from build123d import *

# Parameters (mm, degrees)
EXTRUDE_1_DEPTH = 20
SKETCH_3_W      = 1.25
SKETCH_3_H      = 40.001


with BuildPart() as part:
    # 草图1 → 凸台-拉伸1 (new, symmetric)
    with BuildSketch(Plane(origin=(0, 0, 0), x_dir=(1, 0, 0), z_dir=(0, 1, 0))):
        Polygon((1.327905619, -2.3), (2.655811238, 0), (1.327905619, 2.3), (-1.327905619, 2.3), (-2.655811238, 0), (-1.327905619, -2.3), align=None)
    extrude(amount=EXTRUDE_1_DEPTH, both=True)

    # 草图3 → M3 螺纹孔1 (revolve, cut)
    with BuildSketch(Plane(origin=(0, 20, 0), x_dir=(0, 0, 1), z_dir=(1, 0, 0))):
        with Locations((0.625, 20.0005)):
            Rectangle(SKETCH_3_W, SKETCH_3_H)
    revolve(axis=Axis((0, 26.35, 0), (0, -1, 0)), mode=Mode.SUBTRACT)


solid = part.part
For this review, take the finished solid that the model builds, in its own axes (mm). Give positions to 0.01 mm unless a question says otherwise; leave off trailing zeros. Loops run counter-clockwise (first coordinate to the right, second up) from the corner with the lowest first, then second, coordinate; pieces in that order, holes last.
Item 1: Take a section at C-C, the plane z = 0.4. State the section outline as (x, y) points.
Item 2: Take a section at D-D, the plane x = 2.3. State the section outline as (y, z) points, and give its area (3 significant figures).
Item 3: Draft analysis for pull direction X (two halves, no side actions). For faces 1 (the flat face through (0, 0, 2.3)), 2 (the flat face through (-1.98, 0.28, -1.17)), 3 (the flat face through (1.98, 0.28, 1.17)), 4 (the cylindrical face through (1.22, -0.28, -0.27)), state which applies: +X half, -X half, draft (parallel to the pull), parting line (faces both ways), or undercut.
Item 4: Insertion check: pin 1 (1.5 mm diameter, centred on y = -3, z = 1, fed in from +X); pin 2 (1.5 mm diameter, centred on y = 10, z = -1, fed in from -X). Each pin has a flat end and moves straight along its axis. Give the tip position at first contact, or say it passes through.
Item 5: Take a section at A-A, the plane y = 9. State the section outline as (x, z) points.
Item 6: For line 1 along Z through (x, y) = (0, 4.5); line 2 along X through (y, z) = (-1, 0.6); line 3 along X through (y, z) = (13, -0.1), list the stretches that pass through material, from the lowest coordinate up.
Item 7: Take a section at B-B, the plane x = -0.35. State the section outline as (y, z) points.
Calculated:
1. outline: (-2.42, -20) - (-1.18, -20) - (-1.18, 20) - (-2.42, 20) - close; (1.18, -20) - (2.42, -20) - (2.42, 20) - (1.18, 20) - close
2. outline: (-20, -0.62) - (20, -0.62) - (20, 0.62) - (-20, 0.62) - close
2. area: 49.3 mm2
3. face 1: draft
3. face 2: -X half
3. face 3: +X half
3. face 4: undercut
4. pin 1: stops at x = 2.51
4. pin 2: stops at x = -2.51
5. outline: (-2.66, 0) - (-1.33, -2.3) - (1.33, -2.3) - (2.66, 0) - (1.33, 2.3) - (-1.33, 2.3) - close; hole circle Ø2.5 at (0, 0)
6. line 1: z = -2.3 to -1.25, 1.25 to 2.3
6. line 2: x = -2.31 to -1.1, 1.1 to 2.31
6. line 3: x = -2.6 to -1.25, 1.25 to 2.6
7. outline: (-20, -2.3) - (20, -2.3) - (20, -1.2) - (-20, -1.2) - close; (-20, 1.2) - (20, 1.2) - (20, 2.3) - (-20, 2.3) - close
